Source: CAD feature listing. Evaluate the final solid. Frame: model axes, mm. Round coordinates to 2 decimals unless told otherwise and drop trailing zeros. Write each loop counter-clockwise with the first axis right and the second up, starting at its lowest first coordinate (ties: lowest second). Pieces come first, ordered by that corner, then holes. Notation, with made-up numbers: (-21, -28) -> (34, -28) arc R21 cw to (34, 1) -> close; hole circle Ø4 at (-27.5, -19). An arc over 180 degrees is marked (long way). Put each result on its own line as item: value.
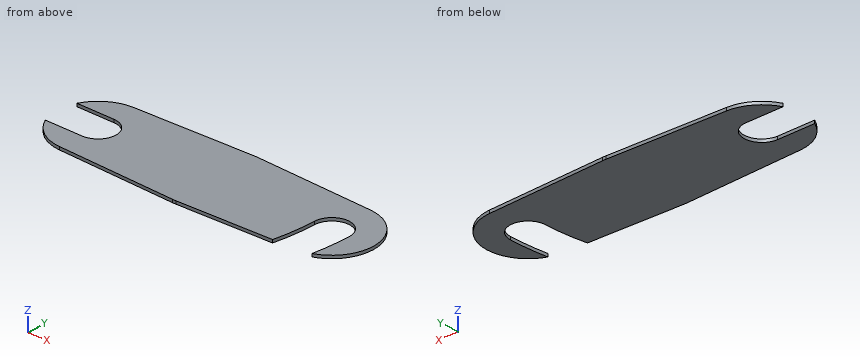
```python
from build123d import *

# Parameters (mm, degrees)
SZKIC1_R                    = 3
DODANIE_WYCI_GNI_CIE1_DEPTH = 0.5
WYTNIJ_WYCI_GNI_CIE1_DEPTH  = 1.5
WYTNIJ_WYCI_GNI_CIE3_DEPTH  = 1.5


with BuildPart() as part:
    # Szkic1 → Dodanie-wyciągnięcie1 (new body)
    with BuildSketch(Plane.XY):
        with BuildLine():
            Line((-0.290625, 7.744548864), (-20.2625, 6.995076393))
            ThreePointArc((-20.2625, 6.995076393), (-27, 0), (-20.2625, -6.995076393))
            Line((-20.2625, -6.995076393), (-0.290625, -7.744548864))
            ThreePointArc((-0.290625, -7.744548864), (0, -7.75), (0.290625, -7.744548864))
            Line((0.290625, -7.744548864), (20.2625, -6.995076393))
            ThreePointArc((20.2625, -6.995076393), (27, 0), (20.2625, 6.995076393))
            Line((20.2625, 6.995076393), (0.290625, 7.744548864))
            ThreePointArc((0.290625, 7.744548864), (0, 7.75), (-0.290625, 7.744548864))
        make_face()
        with Locations((-20, 0)):
            Circle(SZKIC1_R, mode=Mode.SUBTRACT)
        with Locations((20, 0)):
            Circle(SZKIC1_R, mode=Mode.SUBTRACT)
    extrude(amount=DODANIE_WYCI_GNI_CIE1_DEPTH)

    # Szkic2 → Wytnij-wyciągnięcie1 (cut, through all)
    with BuildSketch(Plane.XY.offset(0.5)):
        with BuildLine():
            Line((-20, 3), (-26.32455532, 3))
            ThreePointArc((-26.32455532, 3), (-27, 0), (-26.32455532, -3))
            Line((-26.32455532, -3), (-20, -3))
            ThreePointArc((-20, -3), (-23, 0), (-20, 3))
        make_face()
    extrude(amount=-WYTNIJ_WYCI_GNI_CIE1_DEPTH, mode=Mode.SUBTRACT)

    # Szkic3 → Wytnij-wyciągnięcie3 (cut, through all)
    with BuildSketch(Plane.XY.offset(0.5)):
        with BuildLine():
            ThreePointArc((17, 0), (16.825547843, -3.588735998), (16.303836429, -7.143630766))
            Line((16.303836429, -7.143630766), (20.2625, -6.995076393))
            ThreePointArc((20.2625, -6.995076393), (21.400000598, -6.858571158), (22.5, -6.538348415))
            ThreePointArc((22.5, -6.538348415), (22.874817784, -3.278719262), (23, 0))
            ThreePointArc((23, 0), (20, -3), (17, 0))
        make_face()
    extrude(amount=-WYTNIJ_WYCI_GNI_CIE3_DEPTH, mode=Mode.SUBTRACT)


solid = part.part
```
Q1. Material intervals for line 1 (X direction, y = -3.75, z = 0.35); line 2 (X direction, y = -0.5, z = 0.4); line 3 (Y direction, x = -18.5, z = 0.4), sorted ascending. Write a range as [from, to].
Ans:
line 1: x = [-25.91, 16.81], [22.84, 25.91]
line 2: x = [-17.04, 17], [23, 26.98]
line 3: y = [-7.06, -2.6], [2.6, 7.06]
Q2. Cut plane A-A on x = -21. Output: boundary loops of the cut face in (y, z), and give its area (3 significant figures).
Ans:
outline: (-6.93, 0) -> (-3, 0) -> (-3, 0.5) -> (-6.93, 0.5) -> close; (3, 0) -> (6.93, 0) -> (6.93, 0.5) -> (3, 0.5) -> close
area: 3.93 mm^2
Q3. Cut plane B-B on z = 0.2. Output: boundary loops of the cut face in (x, y).
Ans:
outline: (-26.32, -3) arc R7 ccw to (-20.26, -7) -> (-0.29, -7.74) arc R7.75 ccw to (0.29, -7.74) -> (16.3, -7.14) arc R37 ccw to (17, 0) arc R3 cw to (23, 0) arc R43 cw to (22.5, -6.54) arc R7 ccw to (20.26, 7) -> (0.29, 7.74) arc R7.75 ccw to (-0.29, 7.74) -> (-20.26, 7) arc R7 ccw to (-26.32, 3) -> (-20, 3) arc R3 cw to (-20, -3) -> close
Q4. Cut plane D-D on x = -8. Output: boundary loops of the cut face in (y, z).
Ans:
outline: (-7.46, 0) -> (7.46, 0) -> (7.46, 0.5) -> (-7.46, 0.5) -> close
Q5. Cut plane C-C on y = -2. Output: boundary loops of the cut face in (x, z), and give its area (3 significant figures).
Ans:
outline: (-17.76, 0) -> (16.95, 0) -> (16.95, 0.5) -> (-17.76, 0.5) -> close; (22.95, 0) -> (26.71, 0) -> (26.71, 0.5) -> (22.95, 0.5) -> close
area: 19.2 mm^2
